The listing builds one solid part. Answer for the finished solid, in the listing's coordinates (mm). Give positions to 0.01 mm unless a question says otherwise; leave off trailing zeros. Answer in a Markdown table with one row per item. Add a question column.
from build123d import *

# Parameters (mm, degrees)
BOX_W         = 28
BOX_H         = 15
BOX_DEPTH     = 1.6
SKETCH_R      = 1.75
SKETCH_R_2    = 1
PAD_DEPTH     = 0.01
SKETCH001_R   = 1
SKETCH001_R_2 = 0.5
POCKET_DEPTH  = 1.611


with BuildPart() as part:
    # Box → Box (new body)
    with BuildSketch(Plane.XY):
        with Locations((14, 7.5)):
            Rectangle(BOX_W, BOX_H)
    extrude(amount=BOX_DEPTH)

    # Sketch → Pad (new body)
    with BuildSketch(Plane.XY.offset(1.6)):
        with Locations((2.4, 2.25)):
            Circle(SKETCH_R)
        with Locations((25.75, 2.25)):
            Circle(SKETCH_R)
        with Locations((2.4, 12.65)):
            Circle(SKETCH_R)
        with Locations((25.75, 12.65)):
            Circle(SKETCH_R)
        with Locations((6.2, 2.45)):
            Circle(SKETCH_R_2)
        with Locations((9, 2.45)):
            Circle(SKETCH_R_2)
        with Locations((18.5, 2.45)):
            Circle(SKETCH_R_2)
        with Locations((22.1, 2.45)):
            Circle(SKETCH_R_2)
    extrude(amount=PAD_DEPTH)

    # Sketch001 → Pocket (cut, through all)
    with BuildSketch(Plane.XY.offset(1.61)):
        with Locations((2.4, 2.25)):
            Circle(SKETCH001_R)
        with Locations((2.4, 12.65)):
            Circle(SKETCH001_R)
        with Locations((25.75, 12.65)):
            Circle(SKETCH001_R)
        with Locations((25.75, 2.25)):
            Circle(SKETCH001_R)
        with Locations((6.2, 2.45)):
            Circle(SKETCH001_R_2)
        with Locations((9, 2.45)):
            Circle(SKETCH001_R_2)
        with Locations((18.5, 2.45)):
            Circle(SKETCH001_R_2)
        with Locations((22.1, 2.45)):
            Circle(SKETCH001_R_2)
    extrude(amount=-POCKET_DEPTH, mode=Mode.SUBTRACT)


solid = part.part
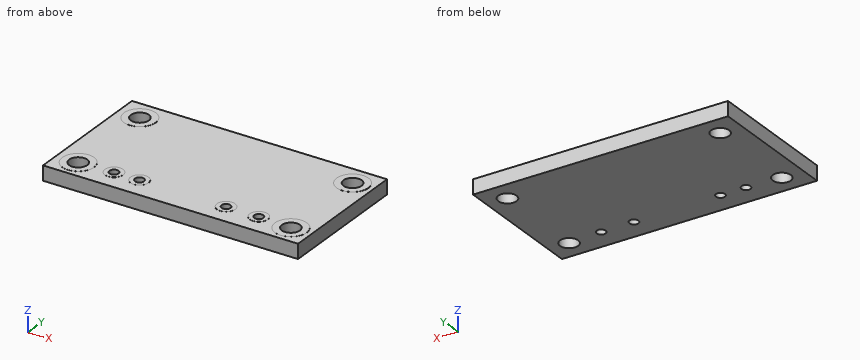
1. Section A-A (z = 1.1) is taken. State how many separate pieces and enclosed holes the cut face has, and give its area (3 significant figures).
2. Straight lines are drawn through the part: L1, parallel to X at y = 3, z = 1.3; L2, parallel to Y at x = 6.2, z = 1.05; L3, parallel to Y at x = 3, z = 0.3. For each, find the intervals that lie inside material, in ascending order. Write a range as [from, to].
3. Given pin 1 Ø2.5 at (x, y) = (2.4, 12.65) entering from +Z, flat-ended and moving along its own axis, determine where the tip first touches the part or whether it passes through.
Geometry check:
| question | item | result |
|---|---|---|
| 1 | separate pieces | 1 |
| 1 | enclosed holes | 8 |
| 1 | area | 404 mm² |
| 2 | L1 | [0, 1.74], [3.06, 25.09], [26.41, 28] |
| 2 | L2 | [0, 1.95], [2.95, 15] |
| 2 | L3 | [0, 1.45], [3.05, 11.85], [13.45, 15] |
| 3 | pin 1 | z = 1.61 |
